Autodesk Inventor part; units mm, degrees
ref_plane "YZ Plane" through (0, 0, 0) normal (1, 0, 0) x (0, 1, 0)
ref_plane "XZ Plane" through (0, 0, 0) normal (0, 1, 0) x (-1, 0, 0)
ref_plane "XY Plane" through (0, 0, 0) normal (0, 0, 1) x (1, 0, 0)
sketch "Эскиз1" plane through (0, 0, 0) normal (0, 0, 1) x (1, 0, 0)
  circle A0 centre (0, 0) radius 4.25
  line L0 (-1.8, 0) -> (1.8, 0) construction
  circle A1 centre (-1.8, 0) radius 0.75
  circle A2 centre (1.8, 0) radius 0.75
  circle A3 centre (0, 0) radius 5.25
  dimension "d0" = 8.5
  dimension "d1" = 3.6
  dimension "d2" = 1.5
  dimension "d3" = 1.5
  dimension "d4" = 1
extrude "Выдавливание1" add sketch "Эскиз1" along normal blind 1 contours A0 | A3
extrude "Выдавливание2" add sketch "Эскиз1" along normal blind 5 from surface at 1 contours A3
properties part number "El_Cap_Support"
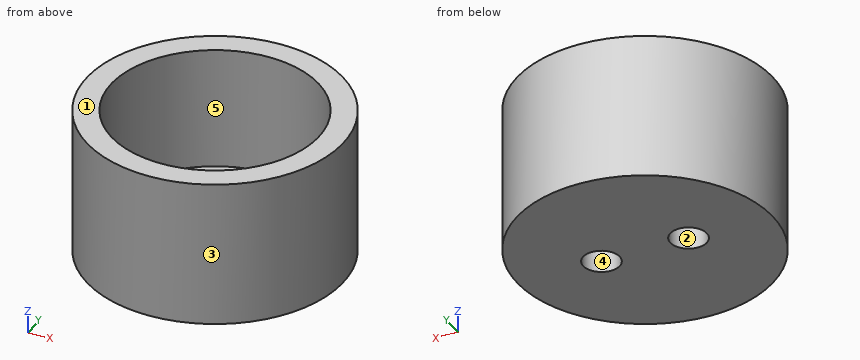
Can you work these out from the model? Positions are in its coordinate system, mm. Face numbers are marked on the shaded views. A direction names the side the tool comes from. Give positions to 0.01 mm unless a question says otherwise; leave off trailing zeros. Loops run counter-clockwise (first coordinate to the right, second up) from the corner with the lowest first, then second, coordinate; pieces in that order, holes last. Notation, with made-up numbers: (6.25, 52.5) - (59.25, 52.5) arc R21 ccw to (59.25, 77.5) - close; hole circle Ø6 at (6, 34). An arc over 180 degrees is marked (long way). Answer as a JSON object with one key per item and string values.
Q1. If we mould it in two halves opening along X, with no side actions, what happens to the marked faces 1, 2 and 3? For each: pulls with the +X half, pulls with the -X half, needs draft (parallel to the pull), parting line crosses it, or undercut.
Geometry says:
{"face 1": "needs draft", "face 2": "undercut", "face 3": "parting line crosses it"}
Q2. If I drill on L1, parallel to Y at x = 0, z = 2.55; L2, parallel to Z at x = -3, y = -2.25; L3, parallel to Y at x = 2.75, z = 1.8, over which ranges is the centre line in solid material (lowest first)?
Geometry says:
{"L1": "-5.25 to -4.25, 4.25 to 5.25", "L2": "0 to 1", "L3": "-4.47 to -3.24, 3.24 to 4.47"}
Q3. Will these pins go through, and if not, where does the flat tip stop? P1, Ø1.5, axis at y = 1, z = 2, coming from the +X side; P2, Ø2, axis at x = 2, z = 3, coming from the +Y side; P3, Ø2.5, axis at x = 1, y = -0.5, coming from the +Z side; P4, Ø1.4, axis at x = -1.8, y = 0, coming from the -Z side.
Geometry says:
{"P1": "x = 5.24", "P2": "y = 5.15", "P3": "z = 1", "P4": "through"}
Q4. Imagine slicing it at A-A on x = 1.5. Write out the boundary of the cut face in (y, z), plus the area to 3 significant figures.
Geometry says:
{"outline": "(-5.03, 0) - (-0.69, 0) - (-0.69, 1) - (-3.98, 1) - (-3.98, 6) - (-5.03, 6) - close; (0.69, 0) - (5.03, 0) - (5.03, 6) - (3.98, 6) - (3.98, 1) - (0.69, 1) - close", "area": "19.2 mm²"}
Q5. Imagine slicing it at B-B on x = 0. Write out the boundary of the cut face in (y, z), plus the area to 3 significant figures.
Geometry says:
{"outline": "(-5.25, 0) - (5.25, 0) - (5.25, 6) - (4.25, 6) - (4.25, 1) - (-4.25, 1) - (-4.25, 6) - (-5.25, 6) - close", "area": "20.5 mm²"}
Q6. Which directions (+Z, -Z, +X, -X, +Y, -Y) give clear straight access to the entire face, cutting with the end or side of a thin tool? Please do the marked faces 4 and 5.
Geometry says:
{"face 4": "+Z, -Z", "face 5": "+Z"}
Q7. Imagine slicing it at D-D on y = 2. Write out the boundary of the cut face in (x, z), plus the area to 3 significant figures.
Geometry says:
{"outline": "(-4.85, 0) - (4.85, 0) - (4.85, 6) - (3.75, 6) - (3.75, 1) - (-3.75, 1) - (-3.75, 6) - (-4.85, 6) - close", "area": "20.7 mm²"}
Q8. Imagine slicing it at C-C on z = 4.95. Write out the boundary of the cut face in (x, y).
Geometry says:
{"outline": "circle Ø10.5 at (0, 0); hole circle Ø8.5 at (0, 0)"}
